Model file for the job. Use its own axes, mm. Coordinates: 2 decimals unless noted, no trailing zeros. Order: outer loops, then holes, each group sorted by start corner. A loop starts at its lowest first (then second) coordinate and runs counter-clockwise, first axis right, second up.
from build123d import *

# Parameters (mm, degrees)
BOSS_EXTRUDE1_DEPTH = 6
FILLET1_R           = 2.54
FILLET2_R           = 1.27
SKETCH2_R           = 1.778
CUT_EXTRUDE1_DEPTH  = 104.544495267


with BuildPart() as part:
    # Sketch1 → Boss-Extrude1 (new body)
    with BuildSketch(Plane.XY):
        Polygon((0, 0), (0, 19.05), (50.8, 19.05), (101.6, 9.525), (101.6, 0), align=None)
    boss_extrude1 = extrude(amount=BOSS_EXTRUDE1_DEPTH)

    # Mirror1: Boss-Extrude1 across plane
    add(boss_extrude1.mirror(Plane(origin=(0, 0, 6), x_dir=(0, 0, 1), z_dir=(1, 0, 0))))

    # Fillet1
    fillet1_edges = [part.edges().sort_by_distance(p)[0] for p in [
        (-101.6, 9.525, 3),
        (101.6, 9.525, 3),
    ]]
    fillet(fillet1_edges, radius=FILLET1_R)

    # Fillet2
    fillet2_edges = [part.edges().sort_by_distance(p)[0] for p in [
        (-101.6, 0, 3),
        (-50.8, 19.05, 3),
        (50.8, 19.05, 3),
        (101.6, 0, 3),
    ]]
    fillet(fillet2_edges, radius=FILLET2_R)

    # Sketch2 → Cut-Extrude1 (cut, through all)
    with BuildSketch(Plane.XY.offset(6)):
        with Locations((-43.8785, 9.525)):
            Circle(SKETCH2_R)
        with Locations((43.8785, 9.525)):
            Circle(SKETCH2_R)
    extrude(amount=-CUT_EXTRUDE1_DEPTH, mode=Mode.SUBTRACT)


solid = part.part
Q1. Cut at A-A, the plane z = 3.65. Count the separate pieces of the cut face and the enclosed holes in it, plus the area to 3 significant figures.
Established:
separate pieces: 1
enclosed holes: 2
area: 3,360 mm2
Q2. Probe line 1 (Y direction, x = -84.5, z = 5.55); line 2 (Y direction, x = 91, z = 1.1). List the from-to ranges inside material, lowest first.
Established:
line 1: y = 0 to 12.73
line 2: y = 0 to 11.51
Q3. Cut at B-B, the plane y = 13.5. List the corners of the cut face in (x, z), plus the area to 3 significant figures.
Established:
outline: (-80.4, 0) - (80.4, 0) - (80.4, 6) - (-80.4, 6) - close
area: 965 mm2
Q4. Cut at C-C, the plane x = 89.5. List the corners of the cut face in (y, z), plus the area to 3 significant figures.
Established:
outline: (0, 0) - (11.79, 0) - (11.79, 6) - (0, 6) - close
area: 70.8 mm2
Q5. Drop a flat-ended pin along its axis: P1, Ø3, axis at x = -43.88, y = 9.52, coming from the -Z side. Give the stop position or say it passes through.
Established:
P1: passes through
Q6. Mould opens along X. For faces 1 (the face through (101.6, 4, 3)), 2 (the face through (-45.655, 9.603, 3.042)), 3 (the face through (42.102, 9.603, 3.042)), 4 (the face through (1, 19.05, 3)) say: pulls with the +X half, pulls with the -X half, needs draft (parallel to the pull), parting line crosses it, or undercut.
Established:
face 1: pulls with the +X half
face 2: undercut
face 3: undercut
face 4: needs draft
